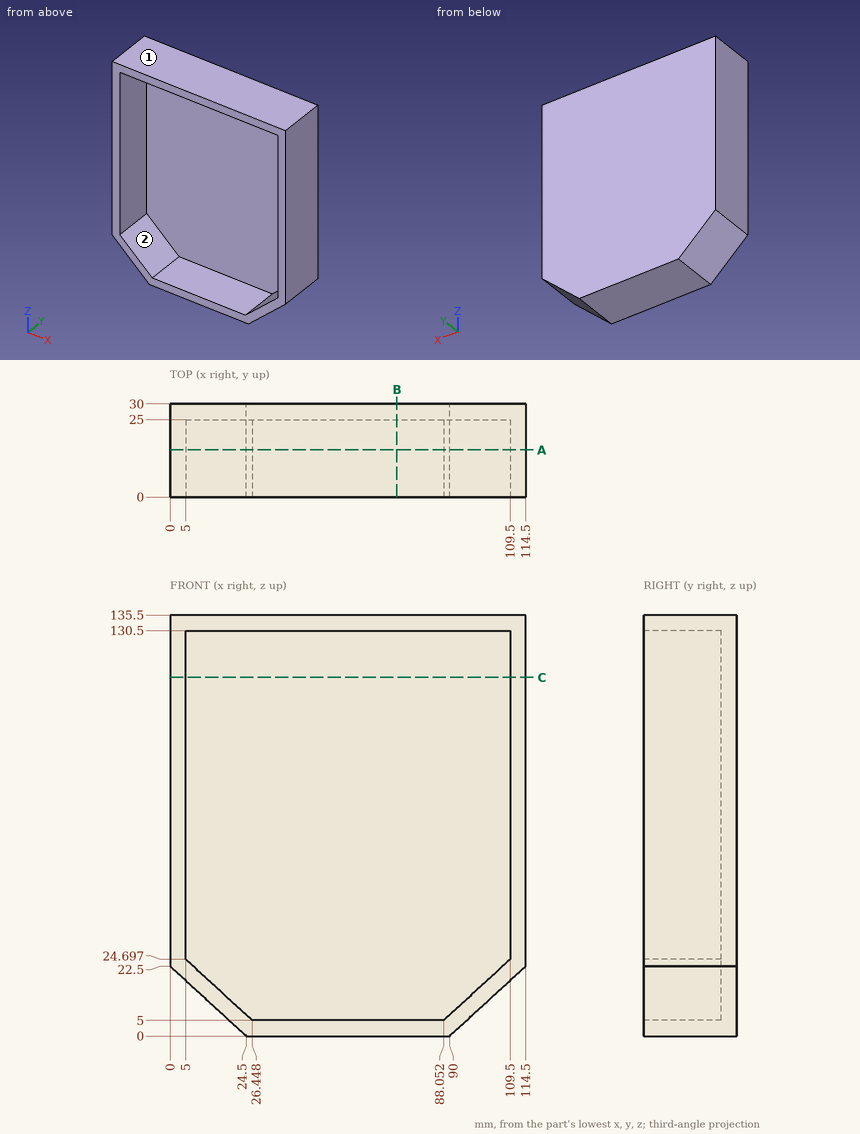
Geometry check sheet. Reference: drawing and pictorial views, mm from the part's lowest x, y, z. A direction names the side the tool comes from. Give positions to 0.01 mm unless a question says otherwise; leave off trailing zeros. Order: outer loops, then holes, each group sorted by start corner. A loop starts at its lowest first (then second) coordinate and runs counter-clockwise, first axis right, second up.
1. Section check C-C, the plane z = 115.5. Enter the section's corners in (x, y).
2. Thickness scan on L1, parallel to Z at x = 31, y = 22; L2, parallel to X at y = 23.75, z = 31; L3, parallel to Y at x = 88, z = 18. Record the ranges inside material, lowest first.
3. Section check B-B, the plane x = 73. Enter the section's corners in (y, z).
4. Section check A-A, the plane y = 15.25. Enter the section's corners in (x, z), and give its area (3 significant figures).
5. Gauge pin test, flat end, axial feed: pin 1 Ø2 at (x, z) = (57.5, 114) entering from -Y. Record the tip position at first contact, or that the pin passes through.
6. Access from +Z, -Z, +X, -X, +Y, -Y to the whole of each face (thin tool, end or side, straight path). Record for the marked faces 1 and 2.
Values follow:
1. outline: (0, 0) - (5, 0) - (5, 25) - (109.5, 25) - (109.5, 0) - (114.5, 0) - (114.5, 30) - (0, 30) - close
2. L1: z = 0 to 5, 130.5 to 135.5
2. L2: x = 0 to 5, 109.5 to 114.5
2. L3: y = 25 to 30
3. outline: (0, 0) - (30, 0) - (30, 135.5) - (0, 135.5) - (0, 130.5) - (25, 130.5) - (25, 5) - (0, 5) - close
4. outline: (0, 22.5) - (24.5, 0) - (90, 0) - (114.5, 22.5) - (114.5, 135.5) - (0, 135.5) - close; hole (5, 24.7) - (26.45, 5) - (88.05, 5) - (109.5, 24.7) - (109.5, 130.5) - (5, 130.5) - close
4. area: 2,270 mm2
5. pin 1: stops at y = 25
6. face 1: +Z, +X, -X, +Y, -Y
6. face 2: -Y
